Read the model definition and answer for the solid it produces. Units are mm, in the model's axes. Give positions to 0.01 mm unless a question says otherwise; leave off trailing zeros. Order: outer loops, then holes, each group sorted by start corner. A loop starts at its lowest first (then second) coordinate and runs counter-clockwise, first axis right, second up.
Item 1: Given pin 1 Ø0.5 at (x, y) = (0, -3) entering from +Z; pin 2 Ø1.3 at (x, z) = (0.5, 0.5) entering from -Y; pin 3 Ø0.7 at (y, z) = (-2.5, 0) entering from +X; pin 4 Ø0.7 at (x, y) = (0, -3) entering from -Z, each flat-ended and moving along its own axis, determine where each tip first touches the part or whether it passes through.
Item 2: A cutting plane is placed at C-C (z = 0.5). Write down the section's boundary in (x, y), plus the area to 3 significant figures.
Item 3: Find the intervals of material crossed by line 1 along X through (y, z) = (-2, -0.05); line 2 along Y through (x, z) = (0.35, 0.35), in increasing order.
Item 4: A cutting plane is placed at B-B (x = -0.55). Write down the section's boundary in (y, z), plus the area to 3 significant figures.
Item 5: A cutting plane is placed at A-A (y = 0.25). Write down the section's boundary in (x, z), plus the area to 3 significant figures.
from build123d import *

# Parameters (mm, degrees)
SKETCH1_W                = 2.54
SKETCH1_H                = 2.54
BOSS_EXTRUDE1_DEPTH      = 3
CHAMFER1_SIZE            = 0.4
BOSS_EXTRUDE2_DEPTH      = 5
BOSS_EXTRUDE2_DEPTH_BACK = 5
SKETCH2_W                = 0.64
SKETCH2_H                = 0.64
SKETCH3_W                = 0.64
SKETCH3_H                = 0.64
BOSS_EXTRUDE3_DEPTH      = 0.5
BOSS_EXTRUDE3_TAPER      = 15


with BuildPart() as part:
    # Sketch1 → Boss-Extrude1 (new body)
    with BuildSketch(Plane(origin=(0, 0, 0), x_dir=(1, 0, 0), z_dir=(0, 1, 0))):
        Rectangle(SKETCH1_W, SKETCH1_H)
    extrude(amount=BOSS_EXTRUDE1_DEPTH)

    # Chamfer1
    chamfer1_edges = [part.edges().sort_by_distance(p)[0] for p in [
        (1.27, 1.5, 1.27),
        (-1.27, 1.5, 1.27),
        (-1.27, 1.5, -1.27),
        (1.27, 1.5, -1.27),
    ]]
    chamfer(chamfer1_edges, length=CHAMFER1_SIZE)

    # Sketch2 → Boss-Extrude2 (add, two sides: drawn at the far end of the back side and taken through both)
    with BuildSketch(Plane.XZ.offset(-BOSS_EXTRUDE2_DEPTH_BACK)):
        Rectangle(SKETCH2_W, SKETCH2_H)
    extrude(amount=BOSS_EXTRUDE2_DEPTH + BOSS_EXTRUDE2_DEPTH_BACK)

    # Sketch3 → Boss-Extrude3 (add)
    with BuildSketch(Plane(origin=(0, 5, 0), x_dir=(1, 0, 0), z_dir=(0, 1, 0))):
        Rectangle(SKETCH3_W, SKETCH3_H)
    boss_extrude3 = extrude(amount=BOSS_EXTRUDE3_DEPTH, taper=BOSS_EXTRUDE3_TAPER)

    # Mirror1: Boss-Extrude3 across plane
    add(boss_extrude3.mirror(Plane.ZX))


solid = part.part
Response values:
1. pin 1: stops at z = 0.32
1. pin 2: stops at y = -5.5
1. pin 3: stops at x = 0.32
1. pin 4: stops at z = -0.32
2. outline: (-1.27, 0) - (1.27, 0) - (1.27, 3) - (-1.27, 3) - close
2. area: 7.62 mm2
3. line 1: x = -0.32 to 0.32
3. line 2: y = 0 to 3
4. outline: (0, -1.27) - (3, -1.27) - (3, 1.27) - (0, 1.27) - close
4. area: 7.62 mm2
5. outline: (-1.27, -0.87) - (-0.87, -1.27) - (0.87, -1.27) - (1.27, -0.87) - (1.27, 0.87) - (0.87, 1.27) - (-0.87, 1.27) - (-1.27, 0.87) - close
5. area: 6.13 mm2
